Can you work these out from the model? Positions are in its coordinate system, mm. A direction names the side the tool comes from. Give positions to 0.01 mm unless a question says otherwise; leave off trailing zeros. Order: outer loops, then holes, each group sorted by start corner. A loop starts at its lowest first (then second) coordinate and runs counter-clockwise, first axis right, second up. Notation, with made-up numbers: M 21,62 L 41,62 A9 ccw 41,74 Z; hole C 9,-16.5 d10. An arc over 180 degrees is marked long. Use one line per item in the form item = value. Start each with the question number.
1. For faces 1 (the face through (11, 3, 0)), 2 (the face through (28.555, 9.86, -10.521)), which set-ups out of +Z, -Z, +X, -X, +Y, -Y let a thin tool reach every point of the face, with its end or its side?
2. I want a section at D-D, the plane x = 31. List the corners of the cut face in (y, z) for me, and give its area (3 significant figures).
3. I need wall thicknesses on L1, parallel to Y at x = 23.5, z = 10; L2, parallel to X at y = 2.3, z = 11.5; L3, parallel to Z at x = 36, y = 19.25. Which ranges of each line are inside material? Lowest first, please.
4. We'd pull the mould along Z, two halves only. Please class faces 3 (the face through (10.1, 1.5, 14.5)), 4 (the face through (31, 20, 5)), 5 (the face through (23.24, 11.62, -12.19)), 6 (the face through (14.4, 2.5, 31.5)): +Z half, -Z half, draft (parallel to the pull), parting line (faces both ways), or undercut.
5. I want a section at A-A, the plane x = 10. List the corners of the cut face in (y, z) for me.
6. I want a section at C-C, the plane y = 13.75. List the corners of the cut face in (x, z) for me, and give its area (3 significant figures).
7. I want a section at B-B, the plane z = -11. List the corners of the cut face in (x, y) for me, and give its area (3 significant figures).
8. Will these pins go through, and if not, where does the flat tip stop? P1, Ø5, axis at y = 14, z = 15, coming from the +X side; P2, Ø10, axis at x = 21.5, z = -11, coming from the -Y side; P3, Ø4, axis at x = 14, y = 7.5, coming from the -Z side; P4, Ø2, axis at y = 6, z = -23, coming from the +X side.
```python
from build123d import *

# Parameters (mm, degrees)
EXTRUDE_1_DEPTH     = 20
CUT_EXTRUDE_1_DEPTH = 17
SKETCH_4_R          = 3
CUT_EXTRUDE_2_DEPTH = 62.491869381


with BuildPart() as part:
    # 草圖2 → 填料-伸長1 (new body)
    with BuildSketch(Plane(origin=(0, 0, 0), x_dir=(1, 0, 0), z_dir=(0, 1, 0))):
        with BuildLine():
            Line((0, 31.5), (20, 31.5))
            ThreePointArc((20, 31.5), (28.786796564, 10.286796564), (50, 1.5))
            Line((50, 1.5), (50, 0))
            Line((50, 0), (0, 0))
            Line((0, 0), (0, 31.5))
        make_face()
    extrude_1 = extrude(amount=EXTRUDE_1_DEPTH)

    # 草圖3 → 除料-伸長1 (cut)
    with BuildSketch(Plane(origin=(0, 20, 0), x_dir=(1, 0, 0), z_dir=(0, 1, 0))):
        with BuildLine():
            Line((0, 31.5), (17, 31.5))
            ThreePointArc((17, 31.5), (23.414353431, 11.949977071), (40.163842214, 0))
            Line((40.163842214, 0), (0, 0))
            Line((0, 0), (0, 31.5))
        make_face()
    cut_extrude_1 = extrude(amount=-CUT_EXTRUDE_1_DEPTH, mode=Mode.SUBTRACT)

    # 草圖4 → 除料-伸長2 (cut, through all)
    with BuildSketch(Plane(origin=(0, 3, 0), x_dir=(1, 0, 0), z_dir=(0, 1, 0))):
        with Locations(Location((10, 11.5, 0), (0, 0, 270))):
            Circle(SKETCH_4_R)
    cut_extrude_2 = extrude(amount=-CUT_EXTRUDE_2_DEPTH, mode=Mode.SUBTRACT)

    # 鏡射4: 填料-伸長1, 除料-伸長1, 除料-伸長2 across plane
    add(extrude_1.mirror(Plane.XY))
    add(cut_extrude_1.mirror(Plane.XY), mode=Mode.SUBTRACT)
    add(cut_extrude_2.mirror(Plane.XY), mode=Mode.SUBTRACT)


solid = part.part
```
Check result:
q1.face_1 = -X, +Y
q1.face_2 = -Z, +X, +Y, -Y
q2.outline = M 0,-8.28 L 20,-8.28 L 20,-4.52 L 3,-4.52 L 3,4.52 L 20,4.52 L 20,8.28 L 0,8.28 Z
q2.area = 178 mm2
q3.L1 = 0 to 3
q3.L2 = 0 to 7, 13 to 27.64
q3.L3 = -4.97 to -1.62, 1.62 to 4.97
q4.face_3 = undercut
q4.face_4 = draft
q4.face_5 = undercut
q4.face_6 = +Z half
q5.outline = M 0,-31.5 L 3,-31.5 L 3,-14.5 L 0,-14.5 Z; M 0,-8.5 L 3,-8.5 L 3,8.5 L 0,8.5 Z; M 0,14.5 L 3,14.5 L 3,31.5 L 0,31.5 Z
q6.outline = M 17,-31.5 L 20,-31.5 A30 cw 50,-1.5 L 50,1.5 A30 cw 20,31.5 L 17,31.5 A33 ccw 40.16,0 A33 ccw Z
q6.area = 277 mm2
q7.outline = M 0,0 L 7.04,0 L 7.04,3 L 0,3 Z; M 12.96,0 L 28.1,0 L 28.1,20 L 24.14,20 L 24.14,3 L 12.96,3 Z
q7.area = 134 mm2
q8.P1 = 26.78
q8.P2 = 0
q8.P3 = through
q8.P4 = 21.54
